For this review, use the dimensioned drawing (mm, ordinates from the lowest corner) and the shaded views. A direction names the side the tool comes from. Give positions to 0.01 mm unless a question says otherwise; leave off trailing zeros. Loops run counter-clockwise (first coordinate to the right, second up) from the corner with the lowest first, then second, coordinate; pieces in that order, holes last. Notation, with made-up numbers: M 62,87 L 69,87 A8 cw 69,99 Z; hole C -30.5,16.25 d11. An arc over 180 degrees is marked long. Use one line per item in the form item = value. Start each with the question number.
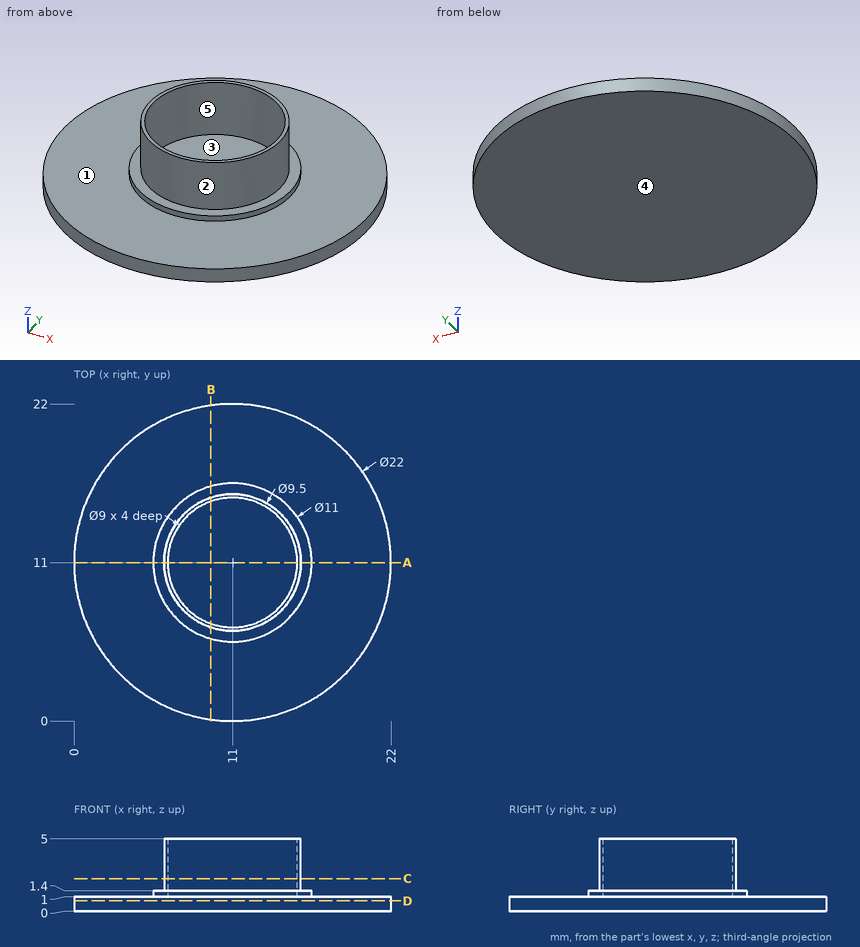
Q1. Take a section at C-C on z = 2.25. Give the boundary of the cut face in (x, y), plus the area to 3 significant figures.
Q2. Clearance check with flat-ended pins moving along their axes: pin 1 Ø4 at (x, y) = (17, 14.5) entering from +Z; pin 2 Ø3 at (x, z) = (8, 1) entering from +Y; pin 3 Ø3.5 at (x, y) = (12.5, 12.5) entering from +Z. State where each tip first meets the part, or that it passes through.
Q3. Take a section at B-B on x = 9.5. Give the boundary of the cut face in (y, z).
Q4. Wall thickness on probe 1 along Y at (x, z) = (11, 2.75); probe 2 along Z at (x, y) = (20, 6.75); probe 3 along X at (y, z) = (12, 2.9): over which ranges is each line inside the solid? List them lowest first.
Q5. The part is to be moulded in two halves that separate along Y. For the marked faces 1, 2 and 3, say which applies: pulls with the +Y half, pulls with the -Y half, needs draft (parallel to the pull), parting line crosses it, or undercut.
Q6. Take a section at A-A on y = 11. Give the boundary of the cut face in (x, z), plus the area to 3 significant figures.
Q7. For the marked faces 4 and 5, list the 3-axis set-ups (+Z, -Z, +X, -X, +Y, -Y) from which the entire face can be reached by the end or side of a thin tool; tool diameter is ignored.
Q8. Take a section at D-D on z = 0.7. Give the boundary of the cut face in (x, y), plus the area to 3 significant figures.
Response values:
q1.outline = C 11,11 d9.5; hole C 11,11 d9
q1.area = 7.26 mm^2
q2.pin_1 = 1.4
q2.pin_2 = 21.9
q2.pin_3 = 1
q3.outline = M 0.1,0 L 21.9,0 L 21.9,1 L 16.29,1 L 16.29,1.4 L 15.51,1.4 L 15.51,5 L 15.24,5 L 15.24,1 L 6.76,1 L 6.76,5 L 6.49,5 L 6.49,1.4 L 5.71,1.4 L 5.71,1 L 0.1,1 Z
q4.probe_1 = 6.25 to 6.5, 15.5 to 15.75
q4.probe_2 = 0 to 1
q4.probe_3 = 6.36 to 6.61, 15.39 to 15.64
q5.face_1 = needs draft
q5.face_2 = parting line crosses it
q5.face_3 = undercut
q6.outline = M 0,0 L 22,0 L 22,1 L 16.5,1 L 16.5,1.4 L 15.75,1.4 L 15.75,5 L 15.5,5 L 15.5,1 L 6.5,1 L 6.5,5 L 6.25,5 L 6.25,1.4 L 5.5,1.4 L 5.5,1 L 0,1 Z
q6.area = 24.6 mm^2
q7.face_4 = -Z, +X, -X, +Y, -Y
q7.face_5 = +Z
q8.outline = C 11,11 d22
q8.area = 380 mm^2
